Can you work these out from the model? Positions are in its coordinate system, mm. Coordinates: 2 decimals unless noted, no trailing zeros. Loops run counter-clockwise (first coordinate to the right, second up) from the corner with the lowest first, then second, coordinate; pieces in that order, holes last.
```python
from build123d import *

# Parameters (mm, degrees)
SKETCH1_R           = 2.5
BOSS_EXTRUDE1_DEPTH = 150
CUT_EXTRUDE1_DEPTH  = 10


with BuildPart() as part:
    # Sketch1 → Boss-Extrude1 (new body)
    with BuildSketch(Plane(origin=(0, 0, 0), x_dir=(1, 0, 0), z_dir=(0, 1, 0))):
        with Locations(Location((0, 0, 0), (0, 0, 270))):
            Circle(SKETCH1_R)
    extrude(amount=BOSS_EXTRUDE1_DEPTH)

    # Sketch5 → Revolve9 (revolve)
    with BuildSketch(Plane(origin=(0, 0, 0), x_dir=(0, 0, -1), z_dir=(1, 0, 0)), mode=Mode.PRIVATE) as revolve9_sk:
        Polygon((-2.75, 150), (0, 150), (0, 153), align=None)
    revolve(revolve9_sk.sketch.rotate(Axis((0, 150, 0), (0, -1, 0)), 180), axis=Axis((0, 150, 0), (0, -1, 0)))

    # Sketch17 → Cut-Extrude1 (cut)
    with BuildSketch(Plane.XZ):
        with BuildLine():
            Line((-2.43587323, 0.605492864), (-1.326757825, -2.130683851))
            ThreePointArc((-1.326757825, -2.130683851), (-2.326158608, -0.94291364), (-2.43587323, 0.605492864))
        make_face()
    extrude(amount=-CUT_EXTRUDE1_DEPTH, mode=Mode.SUBTRACT)

    # Sketch18 → Loft1 section 0
    with BuildSketch(Plane(origin=(0, 0, 0), x_dir=(0, 0, -1), z_dir=(1, 0, 0))):
        with BuildLine():
            Line((2.5, 60), (-2.5, 60))
            Line((-2.5, 60), (-2.5, 64))
            Line((-2.5, 64), (2.5, 64))
            Line((2.5, 64), (2.5, 60))
        make_face()
    # Sketch19 → Loft1 section 1
    with BuildSketch(Plane(origin=(-60, 0, 0), x_dir=(0, 0, -1), z_dir=(1, 0, 0))):
        with BuildLine():
            Line((4.5, 63.668014387), (-2.5, 58))
            Line((-2.5, 58), (-4.5, 60.470000787))
            Line((-4.5, 60.470000787), (2.5, 66.138015175))
            Line((2.5, 66.138015175), (4.5, 63.668014387))
        make_face()
    loft()

    # Sketch20 → Loft2 section 0
    with BuildSketch(Plane(origin=(0, 0, 0), x_dir=(0, 0, -1), z_dir=(1, 0, 0))):
        with BuildLine():
            Line((2.5, 100), (-2.5, 100))
            Line((-2.5, 100), (-2.5, 104))
            Line((-2.5, 104), (2.5, 104))
            Line((2.5, 104), (2.5, 100))
        make_face()
    # Sketch21 → Loft2 section 1
    with BuildSketch(Plane(origin=(60, 0, 0), x_dir=(0, 0, -1), z_dir=(1, 0, 0))):
        with BuildLine():
            Line((-2.5, 106), (-4.5, 103.414213562))
            Line((-4.5, 103.414213562), (2.5, 98))
            Line((2.5, 98), (4.5, 100.585786438))
            Line((4.5, 100.585786438), (-2.5, 106))
        make_face()
    loft()


solid = part.part
```
Item 1: I need wall thicknesses on line 1 along X through (y, z) = (111, 0); line 2 along Y through (x, z) = (-51, 1.5); line 3 along Y through (x, z) = (47.5, -3.25). Which ranges of each line are inside material? Lowest first, please.
Results are:
line 1: x = -2.5 to 2.5
line 2: y = 59.02 to 62.94
line 3: y = 99.78 to 101.84
Item 2: I'm going to push flat-ended pins straight in: P1, Ø2, axis at x = -1.5, y = 68.5, coming from the +Z side; P2, Ø3, axis at y = 91.5, z = -2.5, coming from the -X side; P3, Ø6, axis at x = -7, y = 76, coming from the -Z side; P4, Ø1.5, axis at x = 1.5, y = 77.5, coming from the -Z side. Where does each tip first touch, or does it pass through?
Results are:
P1: stops at z = 2.45
P2: stops at x = -2.29
P3: passes through
P4: stops at z = -2.38
Item 3: Suppose I cut it at A-A, the plane y = 70. Please give me the cut outline in (x, z), plus the area to 3 significant figures.
Results are:
outline: circle Ø5 at (0, 0)
area: 19.6 mm2
Item 4: We'd pull the mould along Y, two halves only. Please class faces 1 (the face through (2.11, 73.95, 1.34)), 2 (the face through (-60, 62, 0)), 3 (the face through (0, 0, 0)): +Y half, -Y half, draft (parallel to the pull), parting line (faces both ways), or undercut.
Results are:
face 1: undercut
face 2: draft
face 3: -Y half
